Could you check a few things on this model? Use its own coordinates, in mm. A direction names the side the tool comes from. Coordinates: 2 decimals unless noted, no trailing zeros. Loops run counter-clockwise (first coordinate to the right, second up) from the corner with the lowest first, then second, coordinate; pieces in that order, holes last. Notation, with made-up numbers: M 69.5,5.25 L 73.5,5.25 A19 cw 73.5,13.25 Z; hole C 29.5,20 d4. An arc over 180 degrees is marked long. Use one line per item in the form item = value. Start each with the question number.
```python
from build123d import *

# Parameters (mm, degrees)
SKETCH1_W           = 127
SKETCH1_H           = 127
BOSS_EXTRUDE1_DEPTH = 127
SKETCH2_W           = 76.2
SKETCH2_H           = 76.2
CUT_EXTRUDE1_DEPTH  = 156.542598667
CHAMFER1_SIZE       = 2.54
FILLET1_R           = 6.35


with BuildPart() as part:
    # Sketch1 → Boss-Extrude1 (new body)
    with BuildSketch(Plane(origin=(0, 0, 0), x_dir=(1, 0, 0), z_dir=(0, 1, 0))):
        Rectangle(SKETCH1_W, SKETCH1_H)
    extrude(amount=BOSS_EXTRUDE1_DEPTH)

    # Sketch2 → Cut-Extrude1 (cut, through all)
    with BuildSketch(Plane(origin=(0, 127, 0), x_dir=(1, 0, 0), z_dir=(0, 1, 0))):
        Rectangle(SKETCH2_W, SKETCH2_H)
    extrude(amount=-CUT_EXTRUDE1_DEPTH, mode=Mode.SUBTRACT)

    # Chamfer1
    chamfer1_edges = [part.edges().sort_by_distance(p)[0] for p in [
        (0, 0, 38.1),
        (-38.1, 0, 0),
        (0, 0, -38.1),
        (38.1, 127, 0),
        (0, 127, -38.1),
        (-38.1, 127, 0),
        (0, 127, 38.1),
    ]]
    chamfer(chamfer1_edges, length=CHAMFER1_SIZE)

    # Fillet1
    fillet1_edges = [part.edges().sort_by_distance(p)[0] for p in [
        (-63.5, 127, 0),
        (0, 127, 63.5),
        (63.5, 127, 0),
        (0, 0, 63.5),
        (-63.5, 0, 0),
        (0, 0, -63.5),
        (63.5, 0, 0),
        (0, 127, -63.5),
    ]]
    fillet(fillet1_edges, radius=FILLET1_R)


solid = part.part
```
Item 1: Please list where these lines run through material, in increasing order: line 1 along X through (y, z) = (13.5, 23); line 2 along Y through (x, z) = (56, -57.5).
Item 2: I want a section at B-B (x = -11.5). Write out the boundary of the cut face in (y, z), plus the area to 3 significant figures.
Item 3: I'm going to push a flat-ended pin straight in: P1, Ø5, axis at x = 24.5, z = 37.5, coming from the +Y side. Where does the tip first touch, or does it pass through?
Item 4: For faces 5 (the cylindrical face through (-61.59, 125.19, -0.89)), 6 (the flat face through (-1, 64, -38.1)), which set-ups out of +Z, -Z, +X, -X, +Y, -Y let a thin tool reach every point of the face, with its end or its side?
Item 5: I want a section at A-A (z = -13.5). Write out the boundary of the cut face in (x, y).
Item 6: Thinking about a two-plate mould opening in X: for faces 1 (the flat face through (-1, 63, -63.5)), 2 (the cylindrical face through (61.59, 1.81, -0.89)), 3 (the cylindrical face through (-61.59, 1.81, -0.89)), 4 (the flat face through (-38.1, 64, 1)), which applies, pulls with the +X half, pulls with the -X half, needs draft (parallel to the pull), parting line crosses it, or undercut?
Item 7: I want a section at C-C (y = 15). Write out the boundary of the cut face in (x, z), plus the area to 3 significant figures.
Worked answers:
q1.line_1 = -63.5 to -38.1, 38.1 to 63.5
q1.line_2 = 0.01 to 126.99
q2.outline = M 0,-57.15 A6.35 ccw 6.35,-63.5 L 120.65,-63.5 A6.35 ccw 127,-57.15 L 127,-40.64 L 124.46,-38.1 L 2.54,-38.1 L 0,-40.64 Z; M 0,40.64 L 2.54,38.1 L 124.46,38.1 L 127,40.64 L 127,57.15 A6.35 ccw 120.65,63.5 L 6.35,63.5 A6.35 ccw 0,57.15 Z
q2.area = 6,400 mm²
q3.P1 = 126.36
q4.face_5 = +Z, -Z, -X, +Y
q4.face_6 = +Y, -Y
q5.outline = M -63.5,6.35 A6.35 ccw -57.15,0 L -40.64,0 L -38.1,2.54 L -38.1,124.46 L -40.64,127 L -57.15,127 A6.35 ccw -63.5,120.65 Z; M 38.1,0 L 57.15,0 A6.35 ccw 63.5,6.35 L 63.5,120.65 A6.35 ccw 57.15,127 L 40.64,127 L 38.1,124.46 Z
q6.face_1 = needs draft
q6.face_2 = pulls with the +X half
q6.face_3 = pulls with the -X half
q6.face_4 = undercut
q7.outline = M -63.5,-63.5 L 63.5,-63.5 L 63.5,63.5 L -63.5,63.5 Z; hole M -38.1,-38.1 L 38.1,-38.1 L 38.1,38.1 L -38.1,38.1 Z
q7.area = 10,300 mm²
